Autodesk Inventor part; units mm, degrees
ref_plane "YZ Plane" through (0, 0, 0) normal (1, 0, 0) x (0, 1, 0)
ref_plane "XZ Plane" through (0, 0, 0) normal (0, 1, 0) x (-1, 0, 0)
ref_plane "XY Plane" through (0, 0, 0) normal (0, 0, 1) x (1, 0, 0)
sketch "Sketch1" plane through (0, 0, 0) normal (0, 0, 1) x (1, 0, 0)
  circle A0 centre (0, 0) radius 8.9
  circle A1 centre (0, 0) radius 9.9
  dimension "d0" = 17.8
  dimension "d1" = 19.8
extrude "Extrusion1" add sketch "Sketch1" along normal blind 130
sketch "Sketch2" plane through (0, 0, 0) normal (0, 0, -1) x (-1, 0, 0)
  circle A0 centre (0, 0) radius 9.9
  circle A1 centre (0, 0) radius 4
  dimension "d4" = 8
extrude "Extrusion2" add sketch "Sketch2" along normal blind 2 contours A0 | A1
sketch "Sketch3" plane through (0, 0, 0) normal (0, 0, 1) x (1, 0, 0)
  circle A0 centre (0, 0) radius 4
  dimension "d7" = 8
extrude "Extrusion3" add sketch "Sketch3" along normal blind 5
properties part number "cuerpo"
Input: part model. Units: mm. Frame: model coordinates. A direction names the side the tool comes from. Give positions to 0.01 mm unless a question says otherwise; leave off trailing zeros. Order: outer loops, then holes, each group sorted by start corner. A loop starts at its lowest first (then second) coordinate and runs counter-clockwise, first axis right, second up. Notation, with made-up numbers: (34, 66) -> (67, 66) arc R23 ccw to (67, 74) -> close; hole circle Ø11 at (23.25, 38). An arc over 180 degrees is marked (long way). Use one line per item in the form item = value.
1) Mould query, pull axis Y, two halves, no side actions, for faces 3 (the cylindrical face through (-1.93, 8.69, 64.09)), 4 (the flat face through (0, 0, -2)). Classes: pulls with the +Y half, pulls with the -Y half, needs draft (parallel to the pull), parting line crosses it, or undercut.
Response values:
face_3 = undercut
face_4 = needs draft
2) Section A-A, the plane x = 0. Return loops of the section in (y, z), and give its area (3 significant figures).
Response values:
outline = (-9.9, -2) -> (9.9, -2) -> (9.9, 130) -> (8.9, 130) -> (8.9, 0) -> (4, 0) -> (4, 5) -> (-4, 5) -> (-4, 0) -> (-8.9, 0) -> (-8.9, 130) -> (-9.9, 130) -> close
area = 340 mm^2
3) First-contact query: pin 1 Ø5.5 at (x, y) = (-4, 4) entering from +Z; pin 2 Ø1 at (x, z) = (-7.5, 11.5) entering from -Y; pin 3 Ø1 at (x, z) = (6, 20.5) entering from +Y. Flat tips, straight axial feed; report the tip coordinate or a pass-through.
Response values:
pin_1 = 5
pin_2 = -7
pin_3 = 8.23
4) Reachability of faces 1 (the flat face through (-4, -2, 0)), 2 (the flat face through (-9, 2, 130)) from +Z, -Z, +X, -X, +Y, -Y: full face, straight path, thin tool, end or side. Return the list, or none.
Response values:
face_1 = +Z
face_2 = +Z, +X, -X, +Y, -Y
5) Line query: probe 1 along Y at (x, z) = (0, 84); probe 2 along Z at (x, y) = (-3, 7.25); probe 3 along Z at (x, y) = (-2.5, 2). Output: solid intervals per line, ascending.
Response values:
probe_1 = -9.9 to -8.9, 8.9 to 9.9
probe_2 = -2 to 0
probe_3 = -2 to 5
6) Section D-D, the plane x = -6. Return loops of the section in (y, z), and give its area (3 significant figures).
Response values:
outline = (-7.87, -2) -> (7.87, -2) -> (7.87, 130) -> (6.57, 130) -> (6.57, 0) -> (-6.57, 0) -> (-6.57, 130) -> (-7.87, 130) -> close
area = 370 mm^2
7) Section C-C, the plane z = 28. Return loops of the section in (x, y).
Response values:
outline = circle Ø19.8 at (0, 0); hole circle Ø17.8 at (0, 0)
